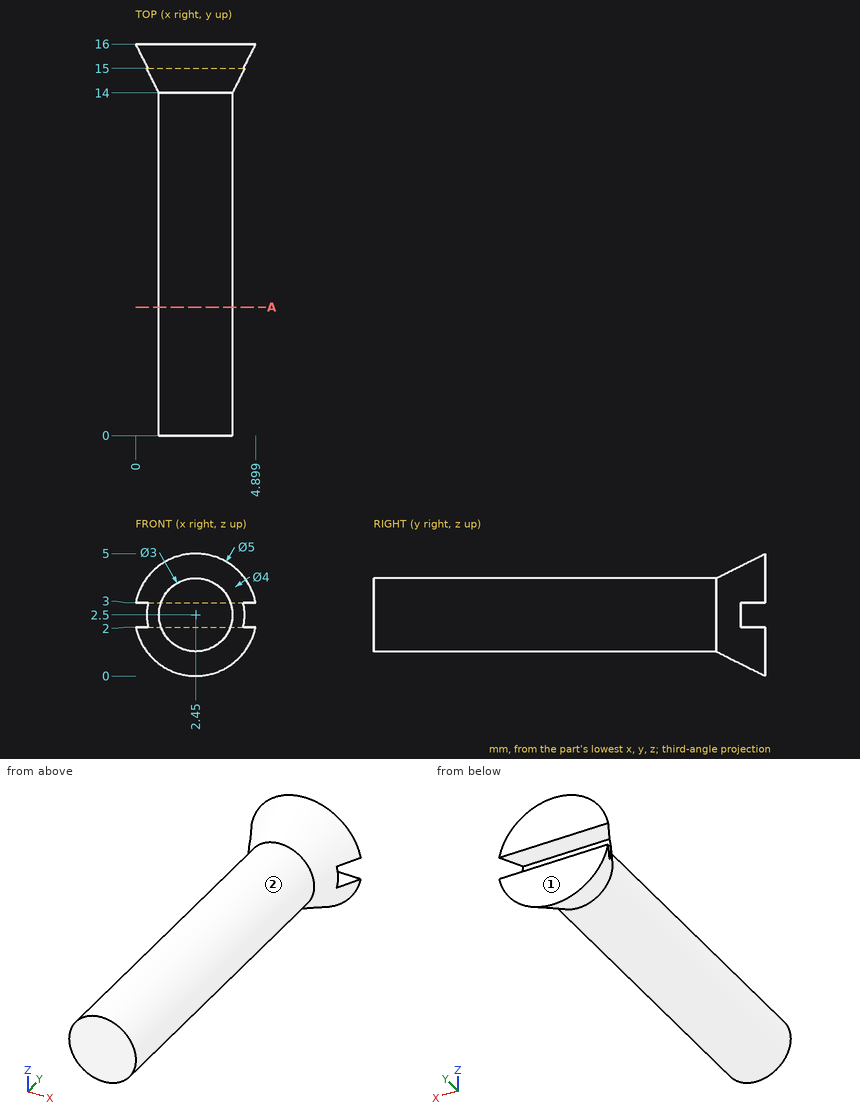
Input: dimensioned drawing with shaded views. Units: mm. Origin: part minimum x, y, z. A direction names the side the tool comes from. Round coordinates to 2 decimals unless told otherwise and drop trailing zeros. Loops run counter-clockwise (first coordinate to the right, second up) from the corner with the lowest first, then second, coordinate; pieces in that order, holes last. Notation, with made-up numbers: (47, 33) -> (96, 33) arc R21 cw to (96, 67) -> close; hole circle Ø10 at (-33.5, 46). An arc over 180 degrees is marked (long way). Use one line per item in the form item = value. Start each with the question number.
1) Access query for the marked faces 1 and 2. Directions: +Z, -Z, +X, -X, +Y, -Y. A direction counts if a zero-diameter tool reaches every point of the face in a straight line with its end or side. Return the directions, or none.
2) Section A-A on y = 5.25. Output: boundary loops of the cut face in (x, z).
3) Line query: L1, parallel to Y at x = 1.9, z = 2.1; L2, parallel to Z at x = 2.4, y = 5.75; L3, parallel to Z at x = 2.85, y = 9.75 (1 decimal). Output: solid intervals per line, ascending.
4) First-contact query: P1, Ø0.5, axis at x = 3.5, z = 2.5, coming from the +Y side; P2, Ø0.5, axis at x = 3, y = 15.5, coming from the +Z side; P3, Ø1, axis at x = 1, y = 3, coming from the -Z side. Flat tips, straight axial feed; report the tip coordinate or a pass-through.
Response:
q1.face_1 = +Z, -Z, +X, -X, +Y
q1.face_2 = -Y
q2.outline = circle Ø3 at (2.45, 2.5)
q3.L1 = 0 to 15
q3.L2 = 1 to 4
q3.L3 = 1.1 to 3.9
q4.P1 = 15
q4.P2 = 4.82
q4.P3 = 1.34
